from build123d import *

# Parameters (mm, degrees)
F1_DEPTH = 25


with BuildPart() as f1:
    # F0 (on Front) → F1 (new body)
    with BuildSketch(Plane.XZ):
        with BuildLine():
            Line((25.196740713, -77.0597371716), (142.969147649, -77.0597371716))
            Line((142.969147649, -77.0597371716), (160.669147649, -77.0597371716))
            Line((160.669147649, -77.0597371716), (160.669147649, -61.3928571429))
            Line((160.669147649, -61.3928571429), (142.969147649, -61.3928571429))
            Line((142.969147649, -61.3928571429), (142.969147649, 153.2071428571))
            Line((142.969147649, 153.2071428571), (160.669147649, 153.2071428571))
            Line((160.669147649, 153.2071428571), (160.669147649, 172.9402628284))
            Line((160.669147649, 172.9402628284), (142.969147649, 172.9402628284))
            Line((142.969147649, 172.9402628284), (21.10726993, 172.9402628284))
            Line((21.10726993, 172.9402628284), (-28.89273007, 172.9402628284))
            Line((-28.89273007, 172.9402628284), (-121.4202080463, 172.9402628284))
            Line((-121.4202080463, 172.9402628284), (-139.1202080463, 172.9402628284))
            Line((-139.1202080463, 172.9402628284), (-139.1202080463, 155.2402628284))
            Line((-139.1202080463, 155.2402628284), (-121.4202080463, 155.2402628284))
            Line((-121.4202080463, 155.2402628284), (-121.8146599785, -59.3593746542))
            Line((-121.8146599785, -59.3593746542), (-139.5146599785, -59.3593746542))
            Line((-139.5146599785, -59.3593746542), (-139.5146599785, -77.0597371716))
            Line((-139.5146599785, -77.0597371716), (-121.630852351, -77.0597371716))
            Line((-121.630852351, -77.0597371716), (-10.803259287, -77.0597371716))
            ThreePointArc((-10.803259287, -77.0597371716), (7.196740713, -59.0597371716), (25.196740713, -77.0597371716))
        make_face()
        with BuildLine():
            Line((-35.2772239302, 38.9654661138), (-44.3083446842, 38.9654661138))
            Line((-44.3083446842, 38.9654661138), (-55.4955438163, 75.4153949225))
            Line((-55.4955438163, 75.4153949225), (-55.7803088852, 75.4153949225))
            add(Edge.make_bspline(
                [(-55.7803088852, 75.4153949225), (-55.1700980234, 64.2993870576), (-55.1700980234, 60.5771008009)],
                knots=[0, 0, 0, 1, 1, 1], degree=2))
            Line((-55.1700980234, 60.5771008009), (-55.1700980234, 38.9654661138))
            Line((-55.1700980234, 38.9654661138), (-63.9774747947, 38.9654661138))
            Line((-63.9774747947, 38.9654661138), (-63.9774747947, 85.4330232363))
            Line((-63.9774747947, 85.4330232363), (-50.5630060172, 85.4330232363))
            Line((-50.5630060172, 85.4330232363), (-39.5690403246, 49.8984107202))
            Line((-39.5690403246, 49.8984107202), (-39.375806885, 49.8984107202))
            Line((-39.375806885, 49.8984107202), (-27.7106092445, 85.4330232363))
            Line((-27.7106092445, 85.4330232363), (-14.306310648, 85.4330232363))
            Line((-14.306310648, 85.4330232363), (-14.306310648, 38.9654661138))
            Line((-14.306310648, 38.9654661138), (-23.4899841174, 38.9654661138))
            Line((-23.4899841174, 38.9654661138), (-23.4899841174, 60.96356768))
            add(Edge.make_bspline(
                [(-23.4899841174, 60.96356768), (-23.4899841174, 62.5196053775), (-23.4391332122, 64.5536415833)],
                knots=[0, 0, 0, 1, 1, 1], degree=2))
            add(Edge.make_bspline(
                [(-23.4391332122, 64.5536415833), (-23.3882823071, 66.5876777892), (-23.011985609, 75.3543738363)],
                knots=[0, 0, 0, 1, 1, 1], degree=2))
            Line((-23.011985609, 75.3543738363), (-23.2967506778, 75.3543738363))
            Line((-23.2967506778, 75.3543738363), (-35.2772239302, 38.9654661138))
        make_face(mode=Mode.SUBTRACT)
        with BuildLine():
            add(Edge.make_bspline(
                [(33.8901772495, 79.9970614762), (39.5651382638, 73.828846682), (39.5651382638, 62.2653508517)],
                knots=[0, 0, 0, 1, 1, 1], degree=2))
            add(Edge.make_bspline(
                [(39.5651382638, 62.2653508517), (39.5651382638, 50.7221953836), (33.8444114349, 44.5234700463)],
                knots=[0, 0, 0, 1, 1, 1], degree=2))
            add(Edge.make_bspline(
                [(33.8444114349, 44.5234700463), (28.1236846059, 38.3247447089), (17.4449945252, 38.3247447089)],
                knots=[0, 0, 0, 1, 1, 1], degree=2))
            add(Edge.make_bspline(
                [(17.4449945252, 38.3247447089), (6.7663044446, 38.3247447089), (1.0455776156, 44.5234700463)],
                knots=[0, 0, 0, 1, 1, 1], degree=2))
            add(Edge.make_bspline(
                [(1.0455776156, 44.5234700463), (-4.6751492133, 50.7221953836), (-4.6751492133, 62.3263719379)],
                knots=[0, 0, 0, 1, 1, 1], degree=2))
            add(Edge.make_bspline(
                [(-4.6751492133, 62.3263719379), (-4.6751492133, 73.9305484922), (1.0608328872, 80.0479123813)],
                knots=[0, 0, 0, 1, 1, 1], degree=2))
            add(Edge.make_bspline(
                [(1.0608328872, 80.0479123813), (6.7968149877, 86.1652762704), (17.5060156114, 86.1652762704)],
                knots=[0, 0, 0, 1, 1, 1], degree=2))
            add(Edge.make_bspline(
                [(17.5060156114, 86.1652762704), (28.2152162352, 86.1652762704), (33.8901772495, 79.9970614762)],
                knots=[0, 0, 0, 1, 1, 1], degree=2))
        make_face(mode=Mode.SUBTRACT)
        Polygon((75.9540459864, 47.1016109372), (75.9540459864, 38.9654661138), (49.1962996985, 38.9654661138), (49.1962996985, 85.4330232363), (75.9540459864, 85.4330232363), (75.9540459864, 77.3578994991), (59.0512051158, 77.3578994991), (59.0512051158, 67.1572079268), (74.784475168, 67.1572079268), (74.784475168, 59.0820841896), (59.0512051158, 59.0820841896), (59.0512051158, 47.1016109372), align=None, mode=Mode.SUBTRACT)
    extrude(amount=F1_DEPTH)


solid = f1.part
Geometry check sheet. Reference: the model listing, model coordinates, mm. A direction names the side the tool comes from. Round coordinates to 2 decimals unless told otherwise and drop trailing zeros. Write each loop counter-clockwise with the first axis right and the second up, starting at its lowest first coordinate (ties: lowest second). Pieces come first, ordered by that corner, then holes.
Item 1: Section check B-B (x = -31.5). Record the boundary of the cut face in (y, z).
Determined:
outline: (-25, -77.06) - (0, -77.06) - (0, 50.44) - (-25, 50.44) - close; (-25, 73.89) - (0, 73.89) - (0, 172.94) - (-25, 172.94) - close
Item 2: Section check A-A (x = 62.5). Record the boundary of the cut face in (y, z), plus the area to 3 significant figures.
Determined:
outline: (-25, -77.06) - (0, -77.06) - (0, 38.97) - (-25, 38.97) - close; (-25, 47.1) - (0, 47.1) - (0, 59.08) - (-25, 59.08) - close; (-25, 67.16) - (0, 67.16) - (0, 77.36) - (-25, 77.36) - close; (-25, 85.43) - (0, 85.43) - (0, 172.94) - (-25, 172.94) - close
area: 5,640 mm2
Item 3: Section check C-C (z = 55). Give the number of separate pieces and of enclosed holes in the cut face, plus the area to 3 significant figures.
Determined:
separate pieces: 7
enclosed holes: 0
area: 4,450 mm2
Item 4: Go/stop test with flat-tipped pins: pin 1 Ø5.5 at (y, z) = (-13, 166.5) entering from -X; pin 2 Ø6.5 at (y, z) = (-11, 46) entering from +X; pin 3 Ø2.5 at (y, z) = (-14.5, 83) entering from -X. Record where each tip stops, or that it passes through.
Determined:
pin 1: stops at x = -139.12
pin 2: stops at x = 142.97
pin 3: stops at x = -121.56
Item 5: Mould release check, pull along Z, two halves, no side actions. Record for faces 5 (the face through (-139.515, -12, -68)), 6 (the face through (75.954, -12, 81)): +Z half, -Z half, draft (parallel to the pull), parting line (faces both ways), or undercut.
Determined:
face 5: draft
face 6: undercut
Item 6: Material ranges on line 1 along Z through (x, y) = (62, -14.5); line 2 along Z through (x, y) = (53.5, -11.5); line 3 along Z through (x, y) = (-122, -3), recorded low to high.
Determined:
line 1: z = -77.06 to 38.97, 47.1 to 59.08, 67.16 to 77.36, 85.43 to 172.94
line 2: z = -77.06 to 38.97, 85.43 to 172.94
line 3: z = -77.06 to -59.36, 155.24 to 172.94
Item 7: Section check D-D (z = -14.5). Record the boundary of the cut face in (x, y).
Determined:
outline: (-121.73, -25) - (142.97, -25) - (142.97, 0) - (-121.73, 0) - close
Item 8: Access from +Z, -Z, +X, -X, +Y, -Y to the whole of each face (thin tool, end or side, straight path). Record for faces 1 (the face through (74.784, -12, 63)), 2 (the face through (152, -12, 153.207)), 3 (the face through (-130, -12, 155.24)), 4 (the face through (160.669, -12, -69)).
Determined:
face 1: +Y, -Y
face 2: +X, +Y, -Y
face 3: -X, +Y, -Y
face 4: +Z, -Z, +X, +Y, -Y
